Check sheet for the modelled part. Datum: model origin and axes. Units: mm. Face numbers are marked on the shaded views. A direction names the side the tool comes from. Give positions to 0.01 mm unless a question says otherwise; leave off trailing zeros. Loops run counter-clockwise (first coordinate to the right, second up) from the corner with the lowest first, then second, coordinate; pieces in that order, holes last. Notation, with made-up numbers: (-33.5, -11) - (-1.5, -11) arc R22 cw to (-1.5, 24) - close; hole circle Ø1 at (10.5, 68). An arc over 180 degrees is marked (long way). Use one line per item in the form item = value.
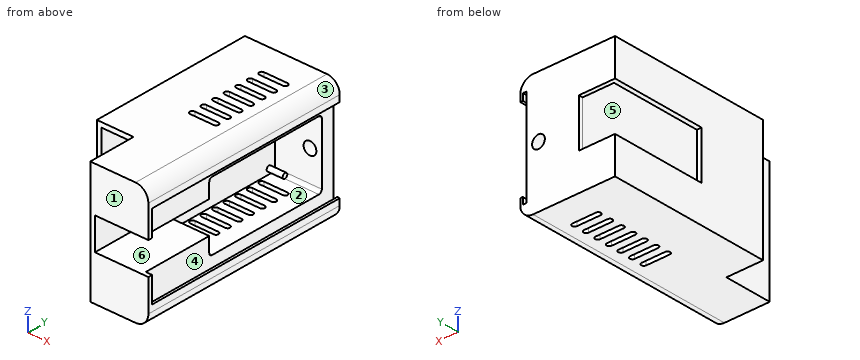
from build123d import *

# Parameters (mm, degrees)
SKETCH1_W                = 37.719
SKETCH1_H                = 84.214152012
BOSS_EXTRUDE1_DEPTH      = 1.905
BOSS_EXTRUDE1_DEPTH_BACK = 46.355
SKETCH3_W                = 14.605
SKETCH3_H                = 19.05
CUT_EXTRUDE1_DEPTH       = 49.26
CUT_EXTRUDE2_DEPTH       = 65.405
CUT_EXTRUDE3_REACH       = 39.719
SKETCH6_W                = 12.7
SKETCH6_H                = 44.45
CUT_EXTRUDE4_DEPTH       = 63.5
CUT_EXTRUDE5_DEPTH       = 21.2471
SKETCH8_R                = 1.016
BOSS_EXTRUDE2_DEPTH      = 6.35
FILLET1_R                = 1.27
CUT_EXTRUDE7_DEPTH       = 82.55
FILLET2_R                = 5.08
CUT_EXTRUDE8_DEPTH       = 38.592
CUT_EXTRUDE8_DEPTH_BACK  = 11.668
CUT_EXTRUDE9_REACH       = 86.214
SKETCH12_R               = 2.54


with BuildPart() as part:
    # Sketch1 → Boss-Extrude1 (new body, two sides)
    with BuildSketch(Plane.XY) as boss_extrude1_sk:
        with Locations((18.8595, -42.107076006)):
            Rectangle(SKETCH1_W, SKETCH1_H)
    extrude(amount=BOSS_EXTRUDE1_DEPTH)
    extrude(boss_extrude1_sk.sketch, amount=-BOSS_EXTRUDE1_DEPTH_BACK)

    # Sketch3 → Cut-Extrude1 (cut, through all)
    with BuildSketch(Plane.XY.offset(1.905)):
        with Locations((7.3025, -74.689152012)):
            Rectangle(SKETCH3_W, SKETCH3_H)
    extrude(amount=-CUT_EXTRUDE1_DEPTH, mode=Mode.SUBTRACT)

    # Sketch4 → Cut-Extrude2 (cut)
    with BuildSketch(Plane(origin=(0, 0, 0), x_dir=(1, 0, 0), z_dir=(0, 1, 0))):
        Polygon((1.905, 22.225), (1.905, 31.75), (14.405235248, 31.75), (14.405235248, 12.7), (1.905, 12.7), align=None)
    extrude(amount=-CUT_EXTRUDE2_DEPTH, mode=Mode.SUBTRACT)

    # Sketch5 → Cut-Extrude3 (cut, up to next)
    with BuildSketch(Plane.ZY, mode=Mode.PRIVATE) as cut_extrude3_sk1:
        Polygon((-22.225, 0), (-12.7, 0), (-12.7, -38.1), (-31.75, -38.1), (-31.75, 0), align=None)
    cut_extrude3_tool1 = extrude(cut_extrude3_sk1.sketch, amount=-CUT_EXTRUDE3_REACH, mode=Mode.PRIVATE) & part.part
    add(cut_extrude3_tool1.solids().sort_by_distance((0, -19.05, -22.225))[0], mode=Mode.SUBTRACT)

    # Sketch6 → Cut-Extrude4 (cut)
    with BuildSketch(Plane.XZ.offset(65.164152012)):
        with Locations((8.255, -22.225)):
            Rectangle(SKETCH6_W, SKETCH6_H)
    extrude(amount=-CUT_EXTRUDE4_DEPTH, mode=Mode.SUBTRACT)

    # Sketch7 → Cut-Extrude5 (cut)
    with BuildSketch(Plane(origin=(37.719, 0, 0), x_dir=(0, 0, -1), z_dir=(1, 0, 0))):
        Polygon((22.225, -5.08), (35.687, -5.08), (35.687, -54.61), (28.575, -54.61), (28.575, -84.214152012), (15.875, -84.214152012), (15.875, -54.61), (8.763, -54.61), (8.763, -5.08), align=None)
    extrude(amount=-CUT_EXTRUDE5_DEPTH, mode=Mode.SUBTRACT)

    # Sketch8 → Boss-Extrude2 (add)
    with BuildSketch(Plane(origin=(16.4719, 0, 0), x_dir=(0, 0, -1), z_dir=(1, 0, 0))):
        with Locations((33.655, -7.62)):
            Circle(SKETCH8_R)
        with Locations((10.795, -7.62)):
            Circle(SKETCH8_R)
    extrude(amount=BOSS_EXTRUDE2_DEPTH)

    # Fillet1
    fillet1_edges = [part.edges().sort_by_distance(p)[0] for p in [
        (27.09545, -5.08, -8.763),
        (27.09545, -5.08, -35.687),
        (27.09545, -54.61, -35.687),
        (27.09545, -54.61, -8.763),
    ]]
    fillet(fillet1_edges, radius=FILLET1_R)

    # Sketch9 → Cut-Extrude7 (cut)
    with BuildSketch(Plane(origin=(0, 0, 0), x_dir=(1, 0, 0), z_dir=(0, 1, 0))):
        Polygon((36.703, 41.402), (35.179, 41.402), (35.179, 3.048), (36.703, 3.048), (36.703, 5.715), (37.719, 5.715), (37.719, 22.225), (37.719, 38.735), (36.703, 38.735), align=None)
    extrude(amount=-CUT_EXTRUDE7_DEPTH, mode=Mode.SUBTRACT)

    # Fillet2
    fillet2_edges = [part.edges().sort_by_distance(p)[0] for p in [
        (37.719, -42.107076006, -46.355),
        (37.719, -42.107076006, 1.905),
    ]]
    fillet(fillet2_edges, radius=FILLET2_R)

    # Sketch10 → Cut-Extrude8 (cut, two sides)
    with BuildSketch(Plane.XY.offset(-35.687)) as cut_extrude8_sk:
        with BuildLine():
            Line((27.559, -13.716), (18.161, -13.716))
            ThreePointArc((18.161, -13.716), (17.145, -12.7), (18.161, -11.684))
            Line((18.161, -11.684), (27.559, -11.684))
            ThreePointArc((27.559, -11.684), (28.575, -12.7), (27.559, -13.716))
        make_face()
        with BuildLine():
            Line((27.559, -18.796), (18.161, -18.796))
            ThreePointArc((18.161, -18.796), (17.145, -17.78), (18.161, -16.764))
            Line((18.161, -16.764), (27.559, -16.764))
            ThreePointArc((27.559, -16.764), (28.575, -17.78), (27.559, -18.796))
        make_face()
        with BuildLine():
            Line((27.559, -23.876), (18.161, -23.876))
            ThreePointArc((18.161, -23.876), (17.145, -22.86), (18.161, -21.844))
            Line((18.161, -21.844), (27.559, -21.844))
            ThreePointArc((27.559, -21.844), (28.575, -22.86), (27.559, -23.876))
        make_face()
        with BuildLine():
            Line((27.559, -28.956), (18.161, -28.956))
            ThreePointArc((18.161, -28.956), (17.145, -27.94), (18.161, -26.924))
            Line((18.161, -26.924), (27.559, -26.924))
            ThreePointArc((27.559, -26.924), (28.575, -27.94), (27.559, -28.956))
        make_face()
        with BuildLine():
            Line((27.559, -34.036), (18.161, -34.036))
            ThreePointArc((18.161, -34.036), (17.145, -33.02), (18.161, -32.004))
            Line((18.161, -32.004), (27.559, -32.004))
            ThreePointArc((27.559, -32.004), (28.575, -33.02), (27.559, -34.036))
        make_face()
        with BuildLine():
            Line((27.559, -39.116), (18.161, -39.116))
            ThreePointArc((18.161, -39.116), (17.145, -38.1), (18.161, -37.084))
            Line((18.161, -37.084), (27.559, -37.084))
            ThreePointArc((27.559, -37.084), (28.575, -38.1), (27.559, -39.116))
        make_face()
        with BuildLine():
            Line((27.559, -44.196), (18.161, -44.196))
            ThreePointArc((18.161, -44.196), (17.145, -43.18), (18.161, -42.164))
            Line((18.161, -42.164), (27.559, -42.164))
            ThreePointArc((27.559, -42.164), (28.575, -43.18), (27.559, -44.196))
        make_face()
    extrude(amount=CUT_EXTRUDE8_DEPTH, mode=Mode.SUBTRACT)
    extrude(cut_extrude8_sk.sketch, amount=-CUT_EXTRUDE8_DEPTH_BACK, mode=Mode.SUBTRACT)

    # Sketch12 → Cut-Extrude9 (cut, up to next)
    with BuildSketch(Plane(origin=(0, 0, 0), x_dir=(1, 0, 0), z_dir=(0, 1, 0)), mode=Mode.PRIVATE) as cut_extrude9_sk1:
        with Locations((30.48, 22.225)):
            Circle(SKETCH12_R)
    cut_extrude9_tool1 = extrude(cut_extrude9_sk1.sketch, amount=-CUT_EXTRUDE9_REACH, mode=Mode.PRIVATE) & part.part
    add(cut_extrude9_tool1.solids().sort_by_distance((30.48, 0, -22.225))[0], mode=Mode.SUBTRACT)


solid = part.part
Item 1: Mould release check, pull along Y, two halves, no side actions. Record for the marked faces 1, 2 and 3: released by +Y, released by -Y, zero draft, split by the parting line, or undercut.
Answer block:
face_1 = released by -Y
face_2 = undercut
face_3 = zero draft
Item 2: Section check A-A on z = -17. Record the boundary of the cut face in (x, y) (3 decimals), then the cut area to 3 significant figures.
Answer block:
outline = (0, -65.164) - (1.905, -65.164) - (1.905, -38.1) - (0, -38.1) - close; (14.405, -1.664) - (14.605, -1.664) - (14.605, -84.214) - (16.472, -84.214) - (16.472, -5.08) - (35.179, -5.08) - (35.179, 0) - (14.405, 0) - close
area = 304 mm2
Item 3: Gauge pin test, flat ends, axial feed: P1, Ø2, axis at x = 13.5, z = -5, coming from the -Y side; P2, Ø3, axis at x = 21.5, z = -39, coming from the +Y side; P3, Ø0.8, axis at x = 36, y = -58.5, coming from the +Z side; P4, Ø1, axis at x = 0.5, z = -19, coming from the +Y side. Record the tip position at first contact, or that the pin passes through.
Answer block:
P1 = -1.66
P2 = 0
P3 = 0.95
P4 = -38.1
Item 4: Section check C-C on x = 7. Record the boundary of the cut face in (y, z) (3 decimals), then the cut area to 3 significant figures.
Answer block:
outline = (-65.164, -46.355) - (0, -46.355) - (0, -31.75) - (-1.664, -31.75) - (-1.664, -44.45) - (-65.164, -44.45) - close; (-65.164, 0) - (-1.664, 0) - (-1.664, -12.7) - (0, -12.7) - (0, 1.905) - (-65.164, 1.905) - close
area = 291 mm2
Item 5: Access from +Z, -Z, +X, -X, +Y, -Y to the whole of each face (thin tool, end or side, straight path). Record for the marked faces 4, 5 and 6.
Answer block:
face_4 = +Y
face_5 = -Y
face_6 = +X, -Y
Item 6: Section check D-D on y = -12.7. Give the number of separate pieces and of enclosed holes in the cut face, then the cut area to 3 significant figures.
Answer block:
separate_pieces = 3
enclosed_holes = 0
area = 369 mm2
Item 7: Section check B-B on y = -49.5. Record the boundary of the cut face in (x, z) (3 decimals).
Answer block:
outline = (0, -46.355) - (32.639, -46.355) arc R5.08 ccw to (37.719, -41.275) - (37.719, -38.735) - (36.703, -38.735) - (36.703, -41.402) - (35.179, -41.402) - (35.179, -35.687) - (16.472, -35.687) - (16.472, -8.763) - (35.179, -8.763) - (35.179, -3.048) - (36.703, -3.048) - (36.703, -5.715) - (37.719, -5.715) - (37.719, -3.175) arc R5.08 ccw to (32.639, 1.905) - (0, 1.905) - close; hole (1.905, -44.45) - (14.605, -44.45) - (14.605, 0) - (1.905, 0) - close
Item 8: Thickness scan on L1, parallel to X at y = -40.5, z = -40.5 (3 decimals); L2, parallel to X at y = -50, z = -23.5 (3 decimals); L3, parallel to X at y = -30.5, z = -7 (3 decimals). Record the ranges inside material, lowest first.
Answer block:
L1 = 0 to 1.905, 14.605 to 35.179, 36.703 to 37.719
L2 = 0 to 1.905, 14.605 to 16.472
L3 = 0 to 1.905, 14.605 to 35.179
